```python
from build123d import *

# Parameters (mm, degrees)
SKETCH2_R               = 30
SHELL15_T               = -9
CUT_EXTRUDE2_DEPTH      = 184.113665481
CUT_EXTRUDE2_DEPTH_BACK = 184.113665481
SKETCH4_R               = 1.5


with BuildPart() as part:
    # Sweep1: sweep along a path in Sketch1
    with BuildLine(Plane.XY) as sweep1_path:
        Line((34.976608727, 0), (34.976608727, 70))
        ThreePointArc((34.976608727, 70), (24.725346068, 94.748737342), (-0.023391273, 105))
        Line((-0.023391273, 105), (-120.023391273, 105))
    # Sketch2 → Sweep1 (sweep)
    with BuildSketch(Plane(origin=(0, 0, 0), x_dir=(1, 0, 0), z_dir=(0, 1, 0))):
        with Locations((34.976608727, 0)):
            Circle(SKETCH2_R)
    sweep(path=sweep1_path.line)

    # Shell15
    shell15_openings = [part.faces().sort_by_distance(p)[0] for p in [
        (-120.023391273, 105, 0),
        (34.976608727, 0, 0),
    ]]
    offset(amount=SHELL15_T, openings=shell15_openings, kind=Kind.INTERSECTION)

    # Sketch4 → Cut-Extrude2 (cut, two sides: drawn at the far end of the back side and taken through both)
    with BuildSketch(Plane(origin=(0, 0, 0), x_dir=(0, 0, -1), z_dir=(1, 0, 0)).offset(-CUT_EXTRUDE2_DEPTH_BACK)):
        with Locations((0, 35)):
            Circle(SKETCH4_R)
        with Locations((0, 55)):
            Circle(SKETCH4_R)
        with Locations((0, 15)):
            Circle(SKETCH4_R)
    extrude(amount=CUT_EXTRUDE2_DEPTH + CUT_EXTRUDE2_DEPTH_BACK, mode=Mode.SUBTRACT)


solid = part.part
```
Geometry check sheet. Reference: the model listing, model coordinates, mm. Round coordinates to 2 decimals unless told otherwise and drop trailing zeros. Order: outer loops, then holes, each group sorted by start corner. A loop starts at its lowest first (then second) coordinate and runs counter-clockwise, first axis right, second up. Notation, with made-up numbers: (-14, 16) - (18, 16) arc R12 ccw to (18, 31) - close; hole circle Ø4 at (18.25, 1). An arc over 180 degrees is marked (long way). Use a Markdown table: item, result. Add a question column.
1) Gauge pin test, flat ends, axial feed: P1, Ø6, axis at y = 98, z = 7, coming from the -X side; P2, Ø25, axis at x = 34.98, z = 0, coming from the +Y side; P3, Ø1.8, axis at y = 35, z = 0, coming from the -X side; P4, Ø1, axis at x = 46, z = 5, coming from the +Y side. Record the tip position at first contact, or that the pin passes through.
2) Mould release check, pull along Y, two halves, no side actions. Record for faces 1 (the flat face through (-120.023, 84.6, -6.2)), 2 (the flat face through (28.7, 0, -20.4)), 3 (the cylindrical face through (-60.86, 84.02, -0.92)), 4 (the cylindrical face through (-60.86, 75.03, -1.32)): released by +Y, released by -Y, zero draft, split by the parting line, or undercut.
3) Thickness scan on line 1 along Y through (x, z) = (58, 0); line 2 along Y through (x, z) = (-87.5, -0.5); line 3 along Y through (x, z) = (9.75, 0). Record the ranges inside material, lowest first.
4) Section check A-A (z = -6). Record the cut outline in (x, y), then the cut area to 3 significant figures.
5) Section check C-C (x = -37). Record the cut outline in (y, z).
6) Section check B-B (y = 20.5). Record the cut outline in (x, z).
Established:
| question | item | result |
|---|---|---|
| 1 | P1 | x = 44.68 |
| 1 | P2 | y = 130.98 |
| 1 | P3 | through |
| 1 | P4 | y = 115.82 |
| 2 | face 1 | zero draft |
| 2 | face 2 | released by -Y |
| 2 | face 3 | undercut |
| 2 | face 4 | split by the parting line |
| 3 | line 1 | 0 to 13.5, 16.5 to 33.5, 36.5 to 53.5, 56.5 to 99.3 |
| 3 | line 2 | 75 to 84.01, 125.99 to 135 |
| 3 | line 3 | 0 to 13.5, 16.5 to 33.5, 36.5 to 53.5, 56.5 to 80.02, 125.14 to 134.26 |
| 4 | outline | (-120.02, 75.61) - (-0.02, 75.61) arc R5.61 cw to (5.58, 70) - (5.58, 0) - (14.85, 0) - (14.85, 70) arc R14.88 ccw to (-0.02, 84.88) - (-120.02, 84.88) - close; (-120.02, 125.12) - (-0.02, 125.12) arc R55.12 cw to (55.1, 70) - (55.1, 0) - (64.37, 0) - (64.37, 70) arc R64.39 ccw to (-0.02, 134.39) - (-120.02, 134.39) - close |
| 4 | area | 4,540 mm2 |
| 5 | outline | circle Ø60 at (105, 0); hole circle Ø42 at (105, 0) |
| 6 | outline | circle Ø60 at (34.98, 0); hole circle Ø42 at (34.98, 0) |
